Print and shaded views of the part. All mm, measured from the part's lowest x, y and z. Give positions to 0.01 mm unless a question says otherwise; leave off trailing zeros. Loops run counter-clockwise (first coordinate to the right, second up) from the corner with the lowest first, then second, coordinate; pieces in that order, holes last. Notation, with made-up numbers: M 87.25,62 L 121.25,62 A30 cw 121.25,85 Z; hole C 60,18 d11. An arc over 180 degrees is marked long. Put each result on its own line as item: value. Start each with the question number.
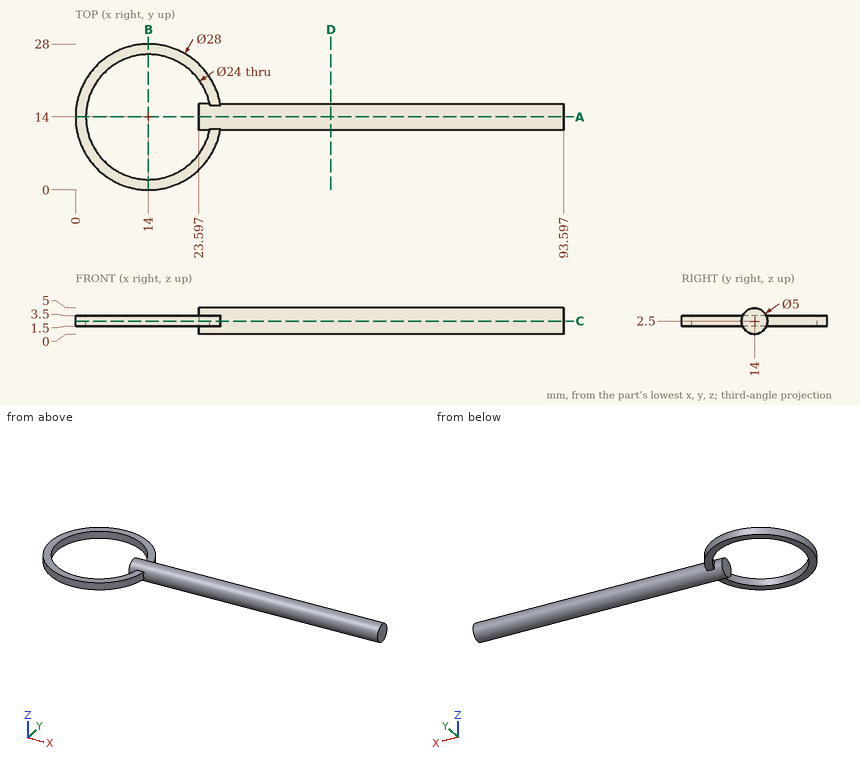
1) Band-saw the part on D-D on x = 49. Give the cut face in (y, z), then the cut area to 3 significant figures.
2) Band-saw the part on C-C on z = 2.5. Give the cut face in (x, y) (1 decimal).
3) Band-saw the part on B-B on x = 14. Give the cut face in (y, z).
4) Band-saw the part on A-A on y = 14. Give the cut face in (x, z).
5) Pin check, flat tips, straight feed: pin 1 Ø8.5 at (x, y) = (15.5, 12.5) entering from +Z; pin 2 Ø1 at (x, z) = (32.5, 3) entering from -Y; pin 3 Ø2 at (y, z) = (19.5, 1) entering from +X. Stop position of each tip, or through.
6) Wall check: L1, parallel to Y at x = 14, z = 2.65; L2, parallel to X at y = 14, z = 2.8; L3, parallel to X at y = 5.5, z = 1.95 (1 decimal). Give the ranges that are in metal, low to high.
Evaluation:
1. outline: C 14,2.5 d5
1. area: 19.6 mm2
2. outline: M 27.8,11.5 L 93.6,11.5 L 93.6,16.5 L 27.8,16.5 A14 ccw long Z; hole M 23.6,11.5 L 23.6,16.5 L 25.7,16.5 A12 ccw long 25.7,11.5 Z
3. outline: M 0,1.5 L 2,1.5 L 2,3.5 L 0,3.5 Z; M 26,1.5 L 28,1.5 L 28,3.5 L 26,3.5 Z
4. outline: M 0,1.5 L 2,1.5 L 2,3.5 L 0,3.5 Z; M 23.6,0 L 93.6,0 L 93.6,5 L 23.6,5 Z
5. pin 1: through
5. pin 2: y = 11.5
5. pin 3: x = 27.21
6. L1: 0 to 2, 26 to 28
6. L2: 0 to 2, 23.6 to 93.6
6. L3: 2.9 to 5.5, 22.5 to 25.1
